Geometry: final body of the model. Coordinates: model frame, mm. Coordinates: 2 decimals unless noted, no trailing zeros. Order: outer loops, then holes, each group sorted by start corner. A loop starts at its lowest first (then second) coordinate and runs counter-clockwise, first axis right, second up. Notation, with made-up numbers: M 43.25,17.5 L 55.25,17.5 A22 ccw 55.25,55.5 Z; hole C -14,17 d10. An arc over 180 degrees is marked long. Use CSV: the item, a comma, the result in double quotes. Start each with the question number.
Q1. First-contact query: P1, Ø0.8, axis at y = 1.5, z = -230.5, coming from the -X side. Flat tip, straight axial feed; report the tip coordinate or a pass-through.
Q2. Section query C-C, the plane z = -32. Output: boundary loops of the cut face in (x, y), and give its area (3 significant figures).
Q3. Section query A-A, the plane y = 1.4. State how many separate pieces and enclosed holes the cut face has, and give its area (3 significant figures).
Q4. Section query B-B, the plane z = -160.5. Output: boundary loops of the cut face in (x, y).
Q5. Ray query, probe 1 along X at (y, z) = (1.15, -112); probe 2 along X at (y, z) = (1.7, -42.5); probe 3 along Z at (x, y) = (-9, 0.3). Return the intervals inside material, ascending.
Autodesk Inventor part; units mm, degrees
ref_plane "YZ Plane" through (0, 0, 0) normal (1, 0, 0) x (0, 1, 0)
ref_plane "XZ Plane" through (0, 0, 0) normal (0, 1, 0) x (-1, 0, 0)
ref_plane "XY Plane" through (0, 0, 0) normal (0, 0, 1) x (1, 0, 0)
sketch "스케치1" plane through (0, 0, 0) normal (0, 1, 0) x (-1, 0, 0)
  line L0 (0, 0) -> (-230, 0)
  line L1 (-230, 0) -> (-230, -309.2)
  line L2 (-230, -309.2) -> (0, -309.2)
  line L3 (0, -309.2) -> (0, 0)
  dimension "d0" = 230
  dimension "d1" = 309.2
extrude "돌출1" add sketch "스케치1" along normal blind 2
sketch "스케치2" plane through (0, 2, 0) normal (0, 1, 0) x (1, 0, 0)
  line L0 (1, 0) -> (1, 309.2)
  line L1 (230, 309.2) -> (0, 309.2)
  line L2 (6.2, 309.2) -> (6.2, 0)
  line L3 (229, 0) -> (229, 309.2)
  line L4 (223.8, 309.2) -> (223.8, 0)
  line L5 (0, 0) -> (230, 0)
  line L6 (0, 309.2) -> (0, 0)
  line L7 (230, 0) -> (230, 309.2)
  line L8 (1, 0) -> (6.2, 0)
  line L9 (1, 309.2) -> (6.2, 309.2)
  line L10 (223.8, 309.2) -> (229, 309.2)
  line L11 (223.8, 0) -> (229, 0)
  dimension "d4" = 1
  dimension "d5" = 5.2
  dimension "d6" = 1
  dimension "d7" = 5.2
extrude "돌출2" cut sketch "스케치2" against normal blind 1 contours L0 L1 L2 L5 | L4 L1 L3 L5
sketch "스케치3" plane through (0, 0, 0) normal (0, -1, 0) x (1, 0, 0)
  line L0 (0, 0) -> (0, -45)
  line L1 (0, -309.2) -> (0, 0)
  line L2 (0, -45) -> (-40, -45)
  line L3 (-40, -45) -> (-40, 0)
  line L4 (-40, 0) -> (0, 0)
  line L5 (230, 0) -> (230, -309.2)
  line L6 (230, 0) -> (230, -45)
  line L7 (230, -45) -> (270, -45)
  line L8 (270, -45) -> (270, 0)
  line L9 (270, 0) -> (230, 0)
  line L10 (230, -309.2) -> (270, -309.2)
  line L11 (270, -309.2) -> (270, -264.2)
  line L12 (270, -264.2) -> (230, -264.2)
  line L13 (0, -309.2) -> (-40, -309.2)
  line L14 (-40, -309.2) -> (-40, -264.2)
  line L15 (-40, -264.2) -> (0, -264.2)
  dimension "d10" = 45
extrude "돌출3" add sketch "스케치3" against normal blind 2
sketch "스케치4" plane through (0, 2, 0) normal (0, 1, 0) x (1, 0, 0)
  line L0 (1, 0) -> (1, 309.2)
  line L1 (1, 309.2) -> (-40, 309.2)
  line L2 (-40, 309.2) -> (-40, 264.2)
  line L3 (-40, 264.2) -> (0, 264.2)
  line L4 (0, 264.2) -> (0, 45)
  line L5 (0, 45) -> (-40, 45)
  line L6 (-40, 45) -> (-40, 0)
  line L7 (-40, 0) -> (1, 0)
  line L8 (223.8, 0) -> (223.8, 309.2)
  line L9 (223.8, 309.2) -> (6.2, 309.2)
  line L10 (6.2, 309.2) -> (6.2, 0)
  line L11 (6.2, 0) -> (223.8, 0)
  line L12 (229, 309.2) -> (229, 0)
  line L13 (229, 0) -> (270, 0)
  line L14 (270, 0) -> (270, 45)
  line L15 (270, 45) -> (230, 45)
  line L16 (230, 45) -> (230, 264.2)
  line L17 (230, 264.2) -> (270, 264.2)
  line L18 (270, 264.2) -> (270, 309.2)
  line L19 (270, 309.2) -> (229, 309.2)
  line L20 (-39, 0) -> (-39, 45)
  line L21 (0, 45) -> (-40, 45)
  line L22 (-33.8, 45) -> (-33.8, 0)
  line L23 (-39, 264.2) -> (-39, 309.2)
  line L24 (1, 309.2) -> (-40, 309.2)
  line L25 (-33.8, 309.2) -> (-33.8, 264.2)
  line L26 (0, 264.2) -> (-40, 264.2)
  line L27 (229, 0) -> (270, 0)
  line L28 (269, 0) -> (269, 45)
  line L29 (230, 45) -> (270, 45)
  line L30 (263.8, 0) -> (263.8, 45)
  line L31 (230, 264.2) -> (270, 264.2)
  line L32 (269, 264.2) -> (269, 309.2)
  line L33 (270, 309.2) -> (229, 309.2)
  line L34 (263.8, 309.2) -> (263.8, 264.2)
  line L35 (263.8, 264.2) -> (269, 264.2)
  line L36 (269, 309.2) -> (263.8, 309.2)
  point P0 (0, 0)
  dimension "d13" = 1
  dimension "d14" = 5.2
  dimension "d15" = 1
  dimension "d16" = 1
  dimension "d17" = 5.2
extrude "돌출4" cut sketch "스케치4" against normal blind 1 contours L7 L20 L5 L22 | L25 L3 L23 L1 | L19 L32 L17 L34 | L30 L15 L28 L13
sketch "스케치5" plane through (0, 2, 0) normal (0, 1, 0) x (1, 0, 0)
  line L0 (223.8, 0) -> (223.8, 309.2)
  line L1 (223.8, 309.2) -> (6.2, 309.2)
  line L2 (6.2, 309.2) -> (6.2, 0)
  line L3 (6.2, 0) -> (223.8, 0)
  line L4 (-33.8, 309.2) -> (-33.8, 264.2)
  line L5 (-33.8, 264.2) -> (0, 264.2)
  line L6 (0, 264.2) -> (0, 45)
  line L7 (0, 45) -> (-33.8, 45)
  line L8 (-33.8, 45) -> (-33.8, 0)
  line L9 (-33.8, 0) -> (1, 0)
  line L10 (1, 0) -> (1, 309.2)
  line L11 (1, 309.2) -> (-33.8, 309.2)
  line L12 (263.8, 0) -> (263.8, 45)
  line L13 (263.8, 45) -> (230, 45)
  line L14 (230, 45) -> (230, 264.2)
  line L15 (230, 264.2) -> (263.8, 264.2)
  line L16 (263.8, 264.2) -> (263.8, 309.2)
  line L17 (263.8, 309.2) -> (229, 309.2)
  line L18 (229, 309.2) -> (229, 0)
  line L19 (229, 0) -> (263.8, 0)
  line L20 (-33.8, 45) -> (-33.8, 0)
  line L21 (-40, 45) -> (0, 45)
  line L22 (-4.8, 24) -> (-4.8, 12)
  line L23 (-5.8, 11) -> (-25.8, 11)
  line L24 (-26.8, 12) -> (-26.8, 24)
  line L25 (-5.8, 25) -> (-25.8, 25)
  line L26 (230, 45) -> (270, 45)
  line L27 (255.8, 25) -> (235.8, 25)
  line L28 (234.8, 24) -> (234.8, 12)
  line L29 (235.8, 11) -> (255.8, 11)
  line L30 (256.8, 12) -> (256.8, 24)
  line L31 (230, 264.2) -> (263.8, 264.2)
  line L32 (255.8, 284.2) -> (235.8, 284.2)
  line L33 (234.8, 285.2) -> (234.8, 297.2)
  line L34 (235.8, 298.2) -> (255.8, 298.2)
  line L35 (256.8, 297.2) -> (256.8, 285.2)
  line L36 (-33.8, 264.2) -> (0, 264.2)
  arc A0 (235.8, 298.2) -> (234.8, 297.2) centre (235.8, 297.2) ccw
  arc A1 (256.8, 297.2) -> (255.8, 298.2) centre (255.8, 297.2) ccw
  arc A2 (255.8, 284.2) -> (256.8, 285.2) centre (255.8, 285.2) ccw
  arc A3 (234.8, 285.2) -> (235.8, 284.2) centre (235.8, 285.2) ccw
  arc A4 (235.8, 25) -> (234.8, 24) centre (235.8, 24) ccw
  arc A5 (234.8, 12) -> (235.8, 11) centre (235.8, 12) ccw
  arc A6 (255.8, 11) -> (256.8, 12) centre (255.8, 12) ccw
  arc A7 (256.8, 24) -> (255.8, 25) centre (255.8, 24) ccw
  arc A8 (-25.8, 25) -> (-26.8, 24) centre (-25.8, 24) ccw
  arc A9 (-26.8, 12) -> (-25.8, 11) centre (-25.8, 12) ccw
  arc A10 (-5.8, 11) -> (-4.8, 12) centre (-5.8, 12) ccw
  arc A11 (-4.8, 24) -> (-5.8, 25) centre (-5.8, 24) ccw
  line L37 (1, 309.2) -> (-33.8, 309.2)
  line L38 (-33.8, 309.2) -> (-26.8, 309.2)
  line L39 (-26.8, 309.2) -> (-26.8, 298.2)
  line L40 (-25.8, 298.2) -> (-5.8, 298.2)
  line L41 (-4.8, 297.2) -> (-4.8, 285.2)
  line L42 (-5.8, 284.2) -> (-25.8, 284.2)
  line L43 (-26.8, 285.2) -> (-26.8, 297.2)
  arc A12 (-5.8, 284.2) -> (-4.8, 285.2) centre (-5.8, 285.2) ccw
  arc A13 (-4.8, 297.2) -> (-5.8, 298.2) centre (-5.8, 297.2) ccw
  arc A14 (-25.8, 298.2) -> (-26.8, 297.2) centre (-25.8, 297.2) ccw
  arc A15 (-26.8, 285.2) -> (-25.8, 284.2) centre (-25.8, 285.2) ccw
  point P0 (0, 0)
  point P1 (-4.8, 11)
  point P2 (234.8, 25)
  point P3 (234.8, 11)
  point P4 (256.8, 11)
  point P5 (234.8, 284.2)
  point P6 (234.8, 298.2)
  point P7 (256.8, 298.2)
  point P8 (-4.8, 284.2)
  point P9 (-4.8, 298.2)
  point P10 (-26.8, 284.2)
  dimension "d27" = 14
  dimension "d29" = 14
  dimension "d33" = 11
  dimension "d34" = 11
  dimension "d35" = 11
  dimension "d37" = 7
  dimension "d38" = 11
  dimension "d39" = 22
  dimension "d40" = 14
  dimension "d41" = 1
  dimension "d42" = 14
extrude "돌출6" cut sketch "스케치5" against normal blind 10 contours L22 A10 L23 A9 L24 A8 L25 A11 | A7 L30 A6 L29 A5 L28 A4 L27 | L32 A3 L33 A0 L34 A1 L35 A2 | L40 A13 L41 A12 L42 A15 L43 A14
properties part number "밑판" material "알루미늄 6061"
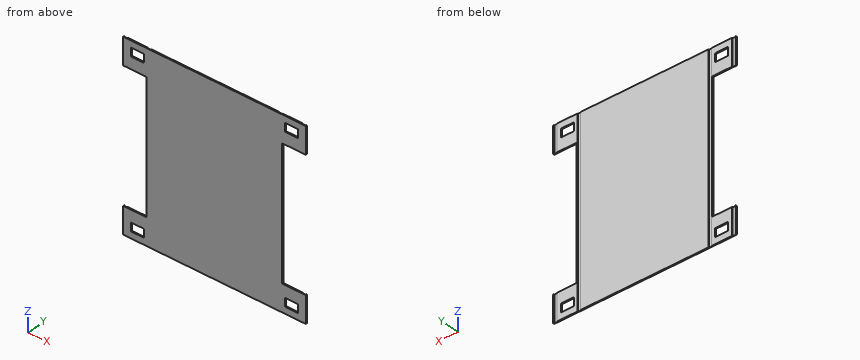
Responses:
1,P1,"stops at x = 0"
2,outline,"M -40,0 L 270,0 L 270,2 L 269,2 L 269,1 L 263.8,1 L 263.8,2 L 229,2 L 229,1 L 223.8,1 L 223.8,2 L 6.2,2 L 6.2,1 L 1,1 L 1,2 L -33.8,2 L -33.8,1 L -39,1 L -39,2 L -40,2 Z"
2,area,"599 mm²"
3,separate pieces,"7"
3,enclosed holes,"4"
3,area,"72,900 mm²"
4,outline,"M 0,0 L 230,0 L 230,2 L 229,2 L 229,1 L 223.8,1 L 223.8,2 L 6.2,2 L 6.2,1 L 1,1 L 1,2 L 0,2 Z"
5,probe 1,"x = 0 to 1, 6.2 to 223.8, 229 to 230"
5,probe 2,"x = -40 to -39, -33.8 to 1, 6.2 to 223.8, 229 to 263.8, 269 to 270"
5,probe 3,"z = -309.2 to -298.2, -284.2 to -264.2, -45 to -25, -11 to 0"
